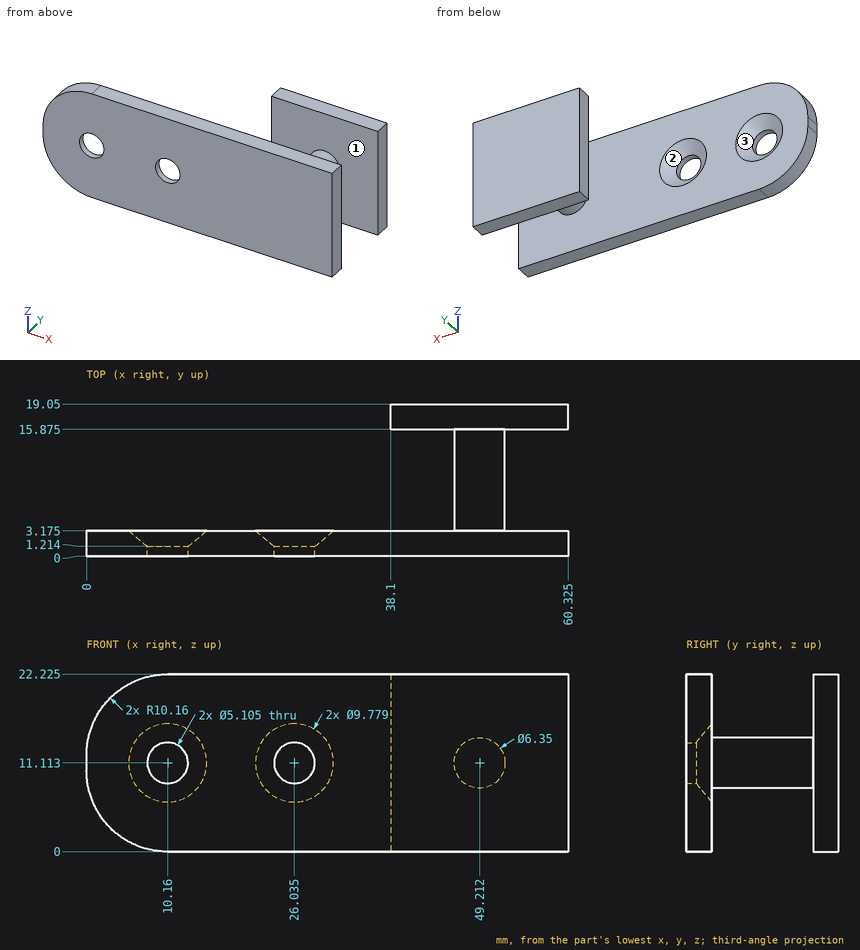
For this review, use the dimensioned drawing (mm, ordinates from the lowest corner) and the shaded views. Round coordinates to 2 decimals unless told otherwise and drop trailing zeros. Use CSV: the item, a comma, the result in double quotes.
1) Wall thickness on line 1 along Z through (x, y) = (10.16, 0.7) (1 decimal); line 2 along Y through (x, z) = (22.5, 19.75) (1 decimal); line 3 along X through (y, z) = (3, 11.25) (1 decimal): over which ranges is each line inside the solid? List them lowest first. Write a range as from..to.
Conclusion:
line 1,"z = 0..8.6, 13.7..22.2"
line 2,"y = 0..3.2"
line 3,"x = 0..5.5, 14.8..21.4, 30.7..60.3"
2) Clearance check with flat-ended pins moving along their axes: pin 1 Ø1 at (y, z) = (17, 12.5) entering from -X; pin 2 Ø5 at (x, z) = (21, 19) entering from +Y (1 decimal); pin 3 Ø3 at (y, z) = (7.5, 13.5) entering from -X (1 decimal). State where each tip first meets the part, or that it passes through.
Conclusion:
pin 1,"stops at x = 38.1"
pin 2,"stops at y = 3.2"
pin 3,"stops at x = 46.2"
3) The part is to be moulded in two halves that separate along Z. For the marked faces 1, 2 and 3, say which applies: pulls with the +Z half, pulls with the -Z half, needs draft (parallel to the pull), parting line crosses it, or undercut.
Conclusion:
face 1,"needs draft"
face 2,"undercut"
face 3,"undercut"
